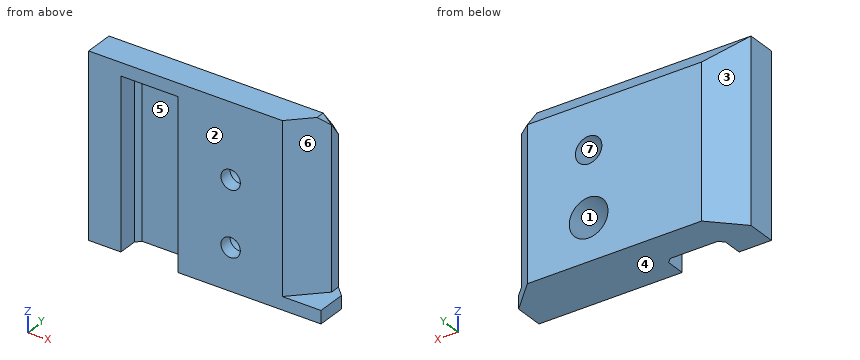
```python
from build123d import *

# Parameters (mm, degrees)
SKETCH1_W               = 36
SKETCH1_H               = 9
BOSS_EXTRUDE1_DEPTH     = 28
CUT_EXTRUDE1_DEPTH      = 28
CUT_EXTRUDE2_DEPTH      = 36
SKETCH5_W               = 11.440376565
SKETCH5_H               = 15.618965423
CUT_EXTRUDE4_DEPTH      = 2
CUT_EXTRUDE5_DEPTH      = 2
CUT_EXTRUDE5_DEPTH_BACK = 2
CUT_EXTRUDE6_DEPTH      = 26
CUT_EXTRUDE7_DEPTH      = 26
SKETCH10_R              = 3
CUT_EXTRUDE8_DEPTH      = 7
SKETCH11_R              = 1.5
CUT_EXTRUDE9_DEPTH      = 2
SKETCH12_R              = 1.5
CUT_EXTRUDE10_DEPTH     = 9
SKETCH13_R              = 2.05
CUT_EXTRUDE11_DEPTH     = 7


with BuildPart() as part:
    # Sketch1 → Boss-Extrude1 (new body)
    with BuildSketch(Plane.XY):
        with Locations((18, 4.5)):
            Rectangle(SKETCH1_W, SKETCH1_H)
    extrude(amount=BOSS_EXTRUDE1_DEPTH)

    # Sketch2 → Cut-Extrude1 (cut)
    with BuildSketch(Plane.XY):
        Polygon((0, 4.5), (4.5, 9), (0, 9), align=None)
        Polygon((36, 4.5), (31.5, 9), (36, 9), align=None)
    extrude(amount=CUT_EXTRUDE1_DEPTH, mode=Mode.SUBTRACT)

    # Sketch3 → Cut-Extrude2 (cut)
    with BuildSketch(Plane(origin=(0, 0, 0), x_dir=(0, 0, -1), z_dir=(1, 0, 0))):
        Polygon((-28, 4.5), (-23.5, 9), (-28, 9), align=None)
    extrude(amount=CUT_EXTRUDE2_DEPTH, mode=Mode.SUBTRACT)

    # Sketch5 → Cut-Extrude4 (cut)
    with BuildSketch(Plane(origin=(32, 0, 32), x_dir=(0, 1, 0), z_dir=(0.707106781, 0, 0.707106781))):
        with Locations((5.720188283, -5.935696583)):
            Rectangle(SKETCH5_W, SKETCH5_H)
    extrude(amount=-CUT_EXTRUDE4_DEPTH, mode=Mode.SUBTRACT)

    # Sketch6 → Cut-Extrude5 (cut, two sides)
    with BuildSketch(Plane(origin=(4, 0, -4), x_dir=(0.577350269, -0.577350269, 0.577350269), z_dir=(-0.707106781, 0, 0.707106781))) as cut_extrude5_sk:
        Polygon((26.558112383, 29.802125204), (32.719347855, 28.647424665), (30.19862658, 32.212262879), align=None)
    extrude(amount=CUT_EXTRUDE5_DEPTH, mode=Mode.SUBTRACT)
    extrude(cut_extrude5_sk.sketch, amount=-CUT_EXTRUDE5_DEPTH_BACK, mode=Mode.SUBTRACT)

    # Sketch7 → Cut-Extrude6 (cut)
    with BuildSketch(Plane.XY):
        Polygon((5, 0), (5, 3), (5.707106781, 3.707106781), (13.104524105, 3.707106781), (13.811630886, 3), (13.811630886, 0), align=None)
    extrude(amount=CUT_EXTRUDE6_DEPTH, mode=Mode.SUBTRACT)

    # Sketch8 → Cut-Extrude7 (cut)
    with BuildSketch(Plane.XY.offset(28)):
        Polygon((36, 0), (30, 0), (34.5, 4.5), (34.5, 6), (36, 6), align=None)
    extrude(amount=-CUT_EXTRUDE7_DEPTH, mode=Mode.SUBTRACT)

    # Sketch10 → Cut-Extrude8 (cut)
    with BuildSketch(Plane(origin=(0, 9, 0), x_dir=(1, 0, 0), z_dir=(0, 1, 0))):
        with Locations((22, -6.5)):
            Circle(SKETCH10_R)
    extrude(amount=-CUT_EXTRUDE8_DEPTH, mode=Mode.SUBTRACT)

    # Sketch11 → Cut-Extrude9 (cut)
    with BuildSketch(Plane(origin=(0, 2, 0), x_dir=(1, 0, 0), z_dir=(0, 1, 0))):
        with Locations((22, -6.5)):
            Circle(SKETCH11_R)
    extrude(amount=-CUT_EXTRUDE9_DEPTH, mode=Mode.SUBTRACT)

    # Sketch12 → Cut-Extrude10 (cut)
    with BuildSketch(Plane(origin=(0, 0, 0), x_dir=(1, 0, 0), z_dir=(0, 1, 0))):
        with Locations((22, -16.5)):
            Circle(SKETCH12_R)
    extrude(amount=CUT_EXTRUDE10_DEPTH, mode=Mode.SUBTRACT)

    # Sketch13 → Cut-Extrude11 (cut)
    with BuildSketch(Plane(origin=(0, 9, 0), x_dir=(1, 0, 0), z_dir=(0, 1, 0))):
        with Locations((22, -16.5)):
            Circle(SKETCH13_R)
    extrude(amount=-CUT_EXTRUDE11_DEPTH, mode=Mode.SUBTRACT)


solid = part.part
```
CAD build for the part. Positions are in the model's coordinates, mm. Face numbers are marked on the shaded views. A direction names the side the tool comes from. Round coordinates to 2 decimals unless told otherwise and drop trailing zeros. Loops run counter-clockwise (first coordinate to the right, second up) from the corner with the lowest first, then second, coordinate; pieces in that order, holes last. Notation, with made-up numbers: M 54,36 L 77,36 A28 cw 77,57 Z; hole C 21,-14 d10. An arc over 180 degrees is marked long. Use a Markdown table: item, result. Add a question column.
(1) Which spindle directions (+Z, -Z, +X, -X, +Y, -Y) get a long thin tool onto all of the face, cutting with end or side? Do the marked faces 4, 5, 6 and 7. Say none if no direction does.
(2) Pull direction X, two halves, no side cores. Call the marked faces 1, 2 and 3: +X half, -X half, draft (parallel to the pull), parting line (faces both ways), or undercut.
(3) Flat gauge pins, fed straight in: pin 1 (5.5 mm diameter, centred on x = 22, z = 16.5, fed in from +Y); pin 2 (1.5 mm diameter, centred on y = 5.5, z = 24.5, fed in from -X); pin 3 (3.5 mm diameter, centred on x = 11, z = 7, fed in from -Y); pin 4 (4 mm diameter, centred on x = 22, z = 6.5, fed in from +Y). Where does each tip first touch, or does it go through?
(4) Drill centre lines: line 1 (Z direction, x = 22, y = 4); line 2 (Z direction, x = 22, y = 1.05); line 3 (X direction, y = 2.5, z = 18). Where is each one in solid material? Low to high.
(5) Cut at D-D (z = 6.5). Give the cut face in (x, y), and give its area (3 significant figures).
(6) Cut at B-B (z = 16.5). Give the cut face in (x, y).
(7) Cut at A-A (x = 22). Give the cut face in (y, z).
(8) Cut at C-C (y = 7.25). Give the cut face in (x, z), and give its area (3 significant figures).
Geometry says:
| question | item | result |
|---|---|---|
| 1 | face 4 | -Z, +X, -X, +Y, -Y |
| 1 | face 5 | -Z, -Y |
| 1 | face 6 | +Z, +X, -Y |
| 1 | face 7 | +Y |
| 2 | face 1 | undercut |
| 2 | face 2 | draft |
| 2 | face 3 | -X half |
| 3 | pin 1 | stops at y = 9 |
| 3 | pin 2 | stops at x = 0.25 |
| 3 | pin 3 | stops at y = 3.71 |
| 3 | pin 4 | stops at y = 2 |
| 4 | line 1 | z = 0 to 3.5, 9.5 to 14.45, 18.55 to 28 |
| 4 | line 2 | z = 0 to 5, 8 to 15, 18 to 28 |
| 4 | line 3 | x = 0 to 5, 13.81 to 20.6, 23.4 to 32.5 |
| 5 | outline | M 0,0 L 5,0 L 5,3 L 5.71,3.71 L 13.1,3.71 L 13.81,3 L 13.81,0 L 20.5,0 L 20.5,2 L 19,2 L 19,9 L 4.5,9 L 0,4.5 Z; M 23.5,0 L 30,0 L 34.5,4.5 L 34.5,6 L 31.5,9 L 25,9 L 25,2 L 23.5,2 Z |
| 5 | area | 206 mm² |
| 6 | outline | M 0,0 L 5,0 L 5,3 L 5.71,3.71 L 13.1,3.71 L 13.81,3 L 13.81,0 L 20.5,0 L 20.5,2 L 19.95,2 L 19.95,9 L 4.5,9 L 0,4.5 Z; M 23.5,0 L 30,0 L 34.5,4.5 L 34.5,6 L 31.5,9 L 24.05,9 L 24.05,2 L 23.5,2 Z |
| 7 | outline | M 0,0 L 9,0 L 9,3.5 L 2,3.5 L 2,5 L 0,5 Z; M 0,8 L 2,8 L 2,9.5 L 9,9.5 L 9,14.45 L 2,14.45 L 2,15 L 0,15 Z; M 0,18 L 2,18 L 2,18.55 L 9,18.55 L 9,23.5 L 4.5,28 L 0,28 Z |
| 8 | outline | M 2.75,0 L 33.25,0 L 33.25,24.15 L 32.15,25.25 L 2.75,25.25 Z; hole C 22,6.5 d6; hole C 22,16.5 d4.1 |
| 8 | area | 728 mm² |
